Here's how the part is built. I have some questions about the finished solid (model axes, mm). A direction names the side the tool comes from. Give positions to 0.01 mm unless a question says otherwise; leave off trailing zeros. Write each loop counter-clockwise with the first axis right and the second up, starting at its lowest first coordinate (ties: lowest second). Pieces come first, ordered by that corner, then holes. Notation, with made-up numbers: M -10,23.25 L 19,23.25 A33 cw 19,54.25 Z; hole C 8,59 d5. An arc over 180 degrees is marked long. Answer as CSV lines item,"result". Start each with the question number.
Q1. Suppose I cut it at A-A (x = 0). Write out the boundary of the cut face in (y, z), then the cut area to 3 significant figures.
Q2. Suppose I cut it at D-D (y = -3.5). Write out the boundary of the cut face in (x, z), then the cut area to 3 significant figures.
Q3. If I drill on line 1 along Y through (x, z) = (0, 0.9); line 2 along Z through (x, y) = (-6.5, -7.5); line 3 along Y through (x, z) = (0.25, 6.25) (3 decimals), over which ranges is the centre line in solid material (lowest first)?
Q4. Suppose I cut it at C-C (y = 0). Write out the boundary of the cut face in (x, z), then the cut area to 3 significant figures.
Q5. For pin 1 (1.5 mm diameter, centred on x = 7.5, y = 6.5, fed in from +Z); pin 2 (8 mm diameter, centred on x = -4, z = 3, fed in from -Y); pin 3 (6 mm diameter, centred on x = -0.5, y = 9, fed in from -Z), each with a flat end and sliding along its axis, tell me the tip position at first contact or that it passes through.
Q6. On a 3-axis mill with a long thin cutter (end or side, diameter ignored), from which of +Z, -Z, +X, -X, +Y, -Y can I reach the whole of each face in a straight line? I mean faces 4 (the cylindrical face through (-8.2, -6.1, 0.6)), 5 (the flat face through (5, -5, 1.2)), 6 (the flat face through (0, 3, 0)). Say none if no direction works.
Q7. Suppose I cut it at B-B (y = 9). Write out the boundary of the cut face in (x, z), then the cut area to 3 significant figures.
Q8. Thinking about a two-plate mould opening in Y: for faces 1 (the flat face through (0, 0, 15)), 2 (the cylindrical face through (0.54, -2.44, -0.74)), 3 (the cylindrical face through (-0.4, 7.4, 0.6)), which applies, +Y half, -Y half, draft (parallel to the pull), parting line (faces both ways), or undercut?
```python
from build123d import *

# Parameters (mm, degrees)
SKETCH1_R           = 12
BOSS_EXTRUDE1_DEPTH = 1.2
SKETCH2_R           = 6.25
BOSS_EXTRUDE2_DEPTH = 13.8
SKETCH3_R           = 1.65
CUT_EXTRUDE1_DEPTH  = 2.2
SKETCH4_R           = 2.5
BOSS_EXTRUDE3_DEPTH = 1.5


with BuildPart() as part:
    # Sketch1 → Boss-Extrude1 (new body)
    with BuildSketch(Plane.XY):
        Circle(SKETCH1_R)
    extrude(amount=BOSS_EXTRUDE1_DEPTH)

    # Sketch2 → Boss-Extrude2 (add)
    with BuildSketch(Plane.XY.offset(1.2)):
        Circle(SKETCH2_R)
    extrude(amount=BOSS_EXTRUDE2_DEPTH)

    # Sketch3 → Cut-Extrude1 (cut, through all)
    with BuildSketch(Plane.XY.offset(1.2)):
        with Locations((0, 9)):
            Circle(SKETCH3_R)
        with Locations((7.794228634, -4.5)):
            Circle(SKETCH3_R)
        with Locations((-7.794228634, -4.5)):
            Circle(SKETCH3_R)
    extrude(amount=-CUT_EXTRUDE1_DEPTH, mode=Mode.SUBTRACT)

    # Sketch4 → Boss-Extrude3 (add)
    with BuildSketch(Plane(origin=(0, 0, 0), x_dir=(-1, 0, 0), z_dir=(0, 0, -1))):
        Circle(SKETCH4_R)
    extrude(amount=BOSS_EXTRUDE3_DEPTH)


solid = part.part
```
Resolved:
1,outline,"M -12,0 L -2.5,0 L -2.5,-1.5 L 2.5,-1.5 L 2.5,0 L 7.35,0 L 7.35,1.2 L 6.25,1.2 L 6.25,15 L -6.25,15 L -6.25,1.2 L -12,1.2 Z; M 10.65,0 L 12,0 L 12,1.2 L 10.65,1.2 Z"
1,area,"205 mm^2"
2,outline,"M -11.48,0 L -9.11,0 L -9.11,1.2 L -11.48,1.2 Z; M -6.48,0 L 6.48,0 L 6.48,1.2 L 5.18,1.2 L 5.18,15 L -5.18,15 L -5.18,1.2 L -6.48,1.2 Z; M 9.11,0 L 11.48,0 L 11.48,1.2 L 9.11,1.2 Z"
2,area,"164 mm^2"
3,line 1,"-12 to 7.35, 10.65 to 12"
3,line 2,"0 to 1.2"
3,line 3,"-6.245 to 6.245"
4,outline,"M -12,0 L -2.5,0 L -2.5,-1.5 L 2.5,-1.5 L 2.5,0 L 12,0 L 12,1.2 L 6.25,1.2 L 6.25,15 L -6.25,15 L -6.25,1.2 L -12,1.2 Z"
4,area,"209 mm^2"
5,pin 1,"z = 1.2"
5,pin 2,"y = -11.99"
5,pin 3,"z = 0"
6,face 4,"+Z, -Z"
6,face 5,"+Z"
6,face 6,"-Z"
7,outline,"M -7.94,0 L -1.65,0 L -1.65,1.2 L -7.94,1.2 Z; M 1.65,0 L 7.94,0 L 7.94,1.2 L 1.65,1.2 Z"
7,area,"15.1 mm^2"
8,face 1,"draft"
8,face 2,"parting line"
8,face 3,"undercut"
